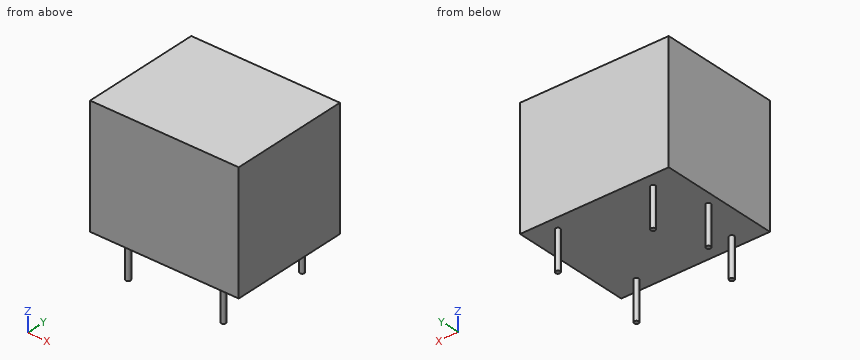
from build123d import *

# Parameters (mm, degrees)
BOX_W     = 19.1
BOX_H     = 15.5
BOX_DEPTH = 15.3
SKETCH_R  = 0.3
PAD_DEPTH = 5
FILLET_R  = 0.1


with BuildPart() as cube:
    # Box → Box (new body)
    with BuildSketch(Plane.XY):
        with Locations((9.55, 7.75)):
            Rectangle(BOX_W, BOX_H)
    extrude(amount=BOX_DEPTH)


with BuildPart() as pad:
    # Pad base: copy of Cube
    add(cube.part)

    # Sketch → Pad (new body)
    with BuildSketch(Plane(origin=(0, 0, 0), x_dir=(1, 0, 0), z_dir=(0, 0, -1))):
        with Locations((1.4, -7.75)):
            Circle(SKETCH_R)
        with Locations((3.45, -1.725)):
            Circle(SKETCH_R)
        with Locations((15.7, -1.725)):
            Circle(SKETCH_R)
        with Locations((3.45, -13.775)):
            Circle(SKETCH_R)
        with Locations((15.7, -13.775)):
            Circle(SKETCH_R)
    extrude(amount=PAD_DEPTH)


with BuildPart() as fillet_body:
    # Fillet base: copy of Pad
    add(pad.part)

    # Fillet
    fillet_edges = [fillet_body.edges().sort_by_distance(p)[0] for p in [
        (9.55, 0, 15.3),
        (0, 7.75, 15.3),
        (9.55, 15.5, 15.3),
        (19.1, 7.75, 15.3),
    ]]
    fillet(fillet_edges, radius=FILLET_R)


with BuildPart() as fusion:
    # Fusion base: copy of Pad
    add(pad.part)

    # Fusion: union Fillet body
    add(fillet_body.part)


with BuildPart() as fusion001:
    # Fusion001 base: copy of Cube
    add(cube.part)

    # Fusion001: union Fusion
    add(fusion.part)


solid = fusion001.part
For this review, take the finished solid that the model builds, in its own axes (mm). Give positions to 0.01 mm unless a question says otherwise; leave off trailing zeros. Loops run counter-clockwise (first coordinate to the right, second up) from the corner with the lowest first, then second, coordinate; pieces in that order, holes last. Notation, with made-up numbers: M 79,8 L 128,8 A17 ccw 128,37 Z; hole C -4,1.5 d4. An arc over 180 degrees is marked long. Put each result on its own line as item: value. Start each with the question number.
(1) Add section D-D, the plane x = 15.7. Write out the cut boundary in (y, z) (3 decimals), then the cut area to 3 significant figures.
(2) Add section A-A, the plane y = 7.75. Write out the cut boundary in (x, z), then the cut area to 3 significant figures.
(3) Wall thickness on L1, parallel to Z at x = 13, y = 9; L2, parallel to X at y = 8, z = -3.5: over which ranges is each line inside the solid? List them lowest first.
(4) For pin 1 (8 mm diameter, centred on x = 13.5, y = 7, fed in from -Z), flat-tipped, find the tip position at first contact; note if it passes through.
(5) Add section C-C, the plane z = -1.5. Write out the cut boundary in (x, y) (3 decimals), then the cut area to 3 significant figures.
(6) Add section B-B, the plane x = 1.4. Write out the cut boundary in (y, z), then the cut area to 3 significant figures.
Result:
1. outline: M 0,0 L 1.425,0 L 1.425,-5 L 2.025,-5 L 2.025,0 L 13.475,0 L 13.475,-5 L 14.075,-5 L 14.075,0 L 15.5,0 L 15.5,15.3 L 0,15.3 Z
1. area: 243 mm^2
2. outline: M 0,0 L 1.1,0 L 1.1,-5 L 1.7,-5 L 1.7,0 L 19.1,0 L 19.1,15.3 L 0,15.3 Z
2. area: 295 mm^2
3. L1: z = 0 to 15.3
3. L2: x = 1.23 to 1.57
4. pin 1: stops at z = 0
5. outline: C 1.4,7.75 d0.6; C 3.45,1.725 d0.6; C 3.45,13.775 d0.6; C 15.7,1.725 d0.6; C 15.7,13.775 d0.6
5. area: 1.41 mm^2
6. outline: M 0,0 L 7.45,0 L 7.45,-5 L 8.05,-5 L 8.05,0 L 15.5,0 L 15.5,15.3 L 0,15.3 Z
6. area: 240 mm^2
